from build123d import *

# Parameters (mm, degrees)
SKETCH_W        = 35
SKETCH_H        = 35
PAD_DEPTH       = 92
SKETCH002_W     = 28
SKETCH002_H     = 28
POCKET001_DEPTH = 89
SKETCH003_W     = 28
SKETCH003_H     = 17
POCKET_DEPTH    = 92.001


with BuildPart() as kegel:
    # Cone → Cone (revolve)
    with BuildSketch(Plane(origin=(0, 19, 0), x_dir=(1, 0, 0), z_dir=(0, 0, -1))):
        Polygon((0, 0), (90, 0), (78, 41), (0, 41), align=None)
    revolve(axis=Axis((0, 19, 0), (0, -1, 0)))


with BuildPart() as cut:
    # Sketch → Pad (new body)
    with BuildSketch(Plane.XY):
        Rectangle(SKETCH_W, SKETCH_H)
    extrude(amount=PAD_DEPTH)

    # Sketch002 → Pocket001 (cut)
    with BuildSketch(Plane.XY):
        Rectangle(SKETCH002_W, SKETCH002_H)
    extrude(amount=POCKET001_DEPTH, mode=Mode.SUBTRACT)

    # Sketch003 → Pocket (cut, through all)
    with BuildSketch(Plane.XY):
        Rectangle(SKETCH003_W, SKETCH003_H)
    extrude(amount=POCKET_DEPTH, mode=Mode.SUBTRACT)

    # Cut: cut Kegel
    add(kegel.part, mode=Mode.SUBTRACT)


solid = cut.part
Design review of the part built by this model. Coordinates are the model's own, in mm. A direction names the side the tool comes from. Round coordinates to 2 decimals unless told otherwise and drop trailing zeros. Write each loop counter-clockwise with the first axis right and the second up, starting at its lowest first coordinate (ties: lowest second). Pieces come first, ordered by that corner, then holes. Notation, with made-up numbers: (19.25, -40) - (65.25, -40) arc R22 cw to (65.25, -8) - close; hole circle Ø3 at (54.25, 58.5). An arc over 180 degrees is marked (long way). Return JSON: item names as keys, results as strings. Group by question number.
Item 1: We need section B-B on y = 11.5. Write out the cut boundary in (x, z).
Item 2: We need section A-A on y = -2. Write out the cut boundary in (x, z).
Item 3: The part is to be moulded in two halves that separate along Y. For faces 4 (the face through (-14, -3, 87)), 5 (the face through (17.5, -4, 86)), 6 (the face through (0.249, -15.801, 79.814)), say which applies: pulls with the +Y half, pulls with the -Y half, needs draft (parallel to the pull), parting line crosses it, or undercut.
Item 4: Insertion check: P1, Ø3, axis at x = 5.5, y = 11.5, coming from the -Z side; P2, Ø10, axis at x = -3.5, y = -12.5, coming from the -Z side. Each pin has a flat end and moves straight along its axis. Give the tip position at first contact, or say it passes through.
Item 5: Machinability: for faces 1 (the face through (0, 17.5, 90)), 2 (the face through (0, 8.5, 90)), 3 (the face through (0, 11, 89)), which of the approach directions +Z, -Z, +X, -X, +Y, -Y give a long, thin tool a straight path to every point of the face, cutting with its end or side? Answer none if there is none.
Item 6: For probe 1 along X at (y, z) = (0, 85.5); probe 2 along Y at (x, z) = (-3.5, 90.5); probe 3 along Y at (x, z) = (-3.5, 84), list the stretches that pass through material, from the lowest coordinate up. Write a range as [from, to].
Model answer:
{
 "1": {"outline": "(-17.5, 86.04) arc R87.8 cw to (-14, 86.68) - (-14, 89) - (14, 89) - (14, 86.68) arc R87.8 cw to (17.5, 86.04) - (17.5, 92) - (-17.5, 92) - close"},
 "2": {"outline": "(-17.5, 82.01) arc R83.85 cw to (-14, 82.68) - (-14, 92) - (-17.5, 92) - close; (14, 82.68) arc R83.85 cw to (17.5, 82.01) - (17.5, 92) - (14, 92) - close"},
 "3": {"face 4": "undercut", "face 5": "needs draft", "face 6": "pulls with the +Y half"},
 "4": {"P1": "stops at z = 89", "P2": "stops at z = 79.22"},
 "5": {"face 1": "+Z, -Z, +X, -X, +Y", "face 2": "+Z, -Z", "face 3": "-Z"},
 "6": {"probe 1": "x = [-17.5, -14], [14, 17.5]", "probe 2": "y = [-17.5, -8.5], [8.5, 17.5]", "probe 3": "y = [-17.5, -14]"}
}
